Can you work these out from the model? Positions are in its coordinate system, mm. A direction names the side the tool comes from. Coordinates: 2 decimals unless noted, no trailing zeros. Loops run counter-clockwise (first coordinate to the right, second up) from the corner with the lowest first, then second, coordinate; pieces in that order, holes last.
```python
from build123d import *

# Parameters (mm, degrees)
F3_DEPTH = 50.8
F4_R     = 5.08
F5_SIZE  = 5.08
F7_W     = 6.725892
F7_H     = 7.135436
F8_DEPTH = 50.8
F9_R     = 1.27


with BuildPart() as f3:
    # F2 (on offset) → F3 (new body)
    with BuildSketch(Plane.XZ.offset(141.478)):
        with BuildLine():
            Line((-111.399229, 60.157929), (-139.718567, 62.847873))
            ThreePointArc((-139.718567, 62.847873), (-128.971224, 25.57843), (-111.399229, 60.157929))
        make_face()
    extrude(amount=F3_DEPTH)

    # F4
    f4_edges = [f3.edges().sort_by_distance(p)[0] for p in [
        (-125.558898, -192.278, 61.502901),
    ]]
    fillet(f4_edges, radius=F4_R)

    # F5
    f5_edges = [f3.edges().sort_by_distance(p)[0] for p in [
        (-128.971224, -141.478, 25.57843),
    ]]
    chamfer(f5_edges, length=F5_SIZE)

    # F7 (on face) → F8 (cut)
    with BuildSketch(Plane(origin=(4.666977, 0, 49.133249), x_dir=(0.995519, 0, -0.094561), z_dir=(0.094561, 0, 0.995519))):
        with Locations((-129.599802, -145.045718)):
            Rectangle(F7_W, F7_H)
    extrude(amount=-F8_DEPTH, mode=Mode.SUBTRACT)

    # F9
    f9_edges = [f3.edges().sort_by_distance(p)[0] for p in [
        (-129.400884, -148.613436, 43.799411),
        (-122.686359, -148.613436, 43.361026),
    ]]
    fillet(f9_edges, radius=F9_R)


solid = f3.part
```
Item 1: I need wall thicknesses on line 1 along X through (y, z) = (-144, 30.5); line 2 along Y through (x, z) = (-123.5, 51.5); line 3 along Z through (x, y) = (-143, -178). Which ranges of each line are inside material? Lowest first, please.
Results are:
line 1: x = -136.16 to -130.66, -123.91 to -117.84
line 2: y = -192.28 to -148.61
line 3: z = 32.97 to 59.69
Item 2: Suppose I cut it at B-B, the plane y = -179. Please give me the cut outline in (x, z).
Results are:
outline: (-139.72, 62.85) arc R20.85 ccw (long way) to (-111.4, 60.16) - close
Item 3: On a 3-axis mill with a long thin cutter (end or side, diameter ignored), from which of +Z, -Z, +X, -X, +Y, -Y can I reach the whole of each face in a straight line? I mean faces 1 (the face through (-125.95, -190.75, 60.085)), 2 (the face through (-126, -148.613, 44)), 3 (the face through (-122.663, -144.452, 43.609)), 4 (the face through (-129.377, -144.452, 44.05)), 5 (the face through (-135, -141.478, 47)). Say none if no direction works.
Results are:
face 1: +Z, +X, -Y
face 2: +Y
face 3: +Z, +Y
face 4: -Z, +Y
face 5: +Z, -Z, +X, -X, +Y
Item 4: We'd pull the mould along X, two halves only. Please class faces 6 (the face through (-118, -141.478, 46)), 7 (the face through (-129.05, -148.25, 43.47)), 8 (the face through (-142.422, -141.725, 42.021)): +X half, -X half, draft (parallel to the pull), parting line (faces both ways), or undercut.
Results are:
face 6: draft
face 7: undercut
face 8: -X half
Item 5: Suppose I cut it at C-C, the plane y = -189. Please give me the cut outline in (x, z), plus the area to 3 significant figures.
Results are:
outline: (-140.09, 62.55) arc R20.85 ccw (long way) to (-111.09, 59.8) - close
area: 1,250 mm2
Item 6: Suppose I cut it at A-A, the plane y = -145. Please give me the cut outline in (x, z).
Results are:
outline: (-137.33, 62.62) arc R19.29 ccw to (-130.95, 27.45) - (-127.7, 61.71) - close; (-124.22, 27.24) arc R19.29 ccw to (-113.79, 60.38) - (-121, 61.07) - close
Item 7: I'm going to push flat-ended pins straight in: P1, Ø3, axis at x = -143.5, y = -169.5, coming from the +Z side; P2, Ø8, axis at x = -131.5, y = -185.5, coming from the -Z side; P3, Ø2, axis at x = -127, y = -155.5, coming from the +Z side; P4, Ø10, axis at x = -111.5, z = 51.5, coming from the +Y side. Where does each tip first touch, or does it pass through?
Results are:
P1: stops at z = 60.81
P2: stops at z = 25.49
P3: stops at z = 61.73
P4: stops at y = -141.48
